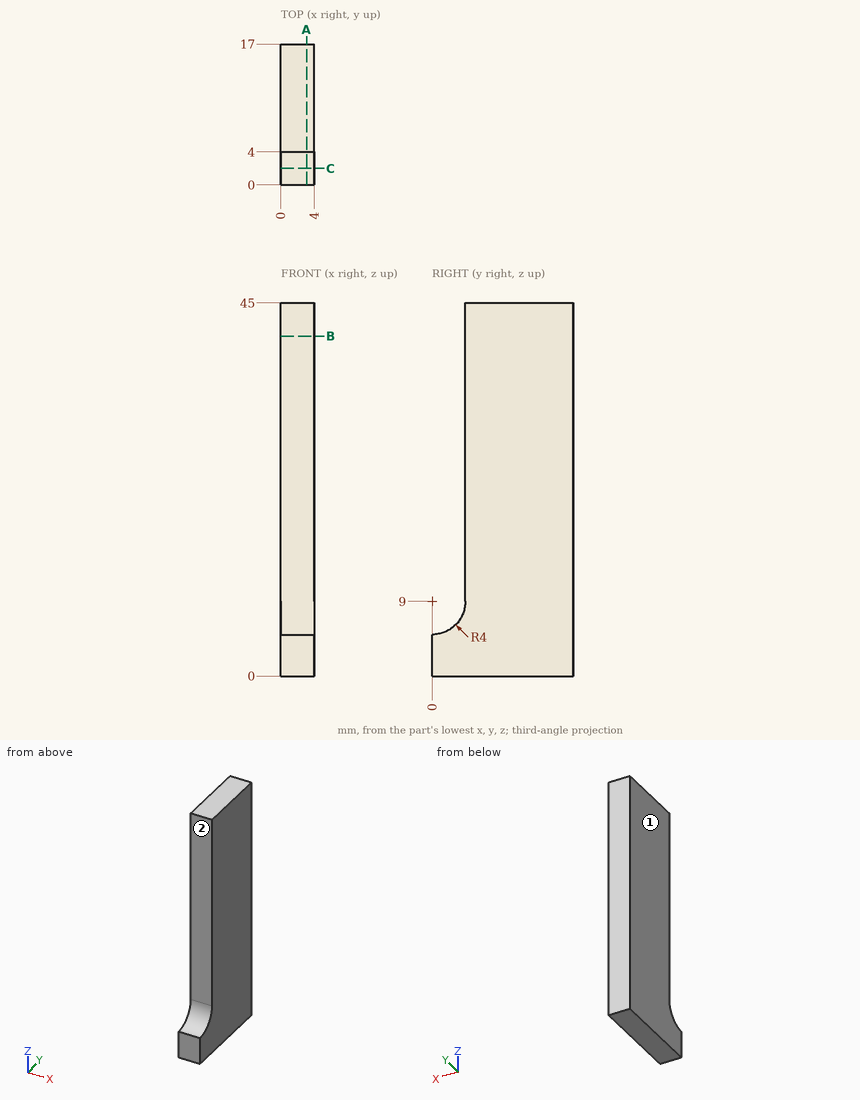
For this review, use the dimensioned drawing (mm, ordinates from the lowest corner) and the shaded views. A direction names the side the tool comes from. Coordinates: 2 decimals unless noted, no trailing zeros. Loops run counter-clockwise (first coordinate to the right, second up) from the corner with the lowest first, then second, coordinate; pieces in that order, holes last. Notation, with made-up numbers: (72, 73.25) -> (124, 73.25) arc R25 cw to (124, 85.25) -> close; hole circle Ø9 at (78, 85). An arc over 180 degrees is marked (long way). Return JSON: item names as keys, results as strings. Group by question number.
(1) Consider section A-A, the plane x = 3.1. Give the boundary of the cut face in (y, z), plus the area to 3 significant figures.
(2) For pin 1 Ø4 at (y, z) = (6.5, 33.5) entering from -X; pin 2 Ø2 at (x, z) = (1, 13.5) entering from -Y, all flat-tipped, find the tip position at first contact; note any pin that passes through.
(3) To check wall thickness, follow L1, parallel to Y at x = 1.4, z = 10; L2, parallel to Y at x = 1.6, z = 8; L3, parallel to Z at x = 3.75, y = 1. State the ranges of each line that lie inside material, in increasing order.
(4) Consider section B-B, the plane z = 41. Give the boundary of the cut face in (x, y), plus the area to 3 significant figures.
(5) Tool access review of the marked faces 1 and 2: name each direction out of +Z, -Z, +X, -X, +Y, -Y from which nothing blocks a thin tool from reaching the whole face with its end or side.
(6) Consider section C-C, the plane y = 2. Give the boundary of the cut face in (x, z).
Results below:
{
 "1": {"outline": "(0, 0) -> (17, 0) -> (17, 45) -> (4, 45) -> (4, 9) arc R4 cw to (0, 5) -> close", "area": "608 mm2"},
 "2": {"pin 1": "stops at x = 0", "pin 2": "stops at y = 4"},
 "3": {"L1": "y = 4 to 17", "L2": "y = 3.87 to 17", "L3": "z = 0 to 5.13"},
 "4": {"outline": "(0, 4) -> (4, 4) -> (4, 17) -> (0, 17) -> close", "area": "52.0 mm2"},
 "5": {"face 1": "+Z, -Z, -X, +Y, -Y", "face 2": "+Z, +X, -X, -Y"},
 "6": {"outline": "(0, 0) -> (4, 0) -> (4, 5.54) -> (0, 5.54) -> close"}
}
